Read the model definition and answer for the solid it produces. Units are mm, in the model's axes. Face numbers are marked on the shaded views. Give positions to 0.01 mm unless a question says otherwise; leave off trailing zeros. Loops run counter-clockwise (first coordinate to the right, second up) from the corner with the lowest first, then second, coordinate; pieces in that order, holes last. Notation, with made-up numbers: M -38.75,-3 L 6.25,-3 A21 ccw 6.25,4 Z; hole C 43,30.25 d7. An arc over 180 degrees is marked long. Return JSON: item names as keys, results as strings. Group by question number.
```python
from build123d import *

# Parameters (mm, degrees)
SKETCH1_R           = 28.5
SKETCH1_R_2         = 23.6
BOSS_EXTRUDE1_DEPTH = 44
SKETCH2_R           = 6
BOSS_EXTRUDE2_DEPTH = 44
SKETCH3_R           = 3.1
CUT_EXTRUDE1_DEPTH  = 45


with BuildPart() as part:
    # Sketch1 → Boss-Extrude1 (new body)
    with BuildSketch(Plane.XY):
        Circle(SKETCH1_R)
        Circle(SKETCH1_R_2, mode=Mode.SUBTRACT)
    extrude(amount=BOSS_EXTRUDE1_DEPTH)

    # Sketch2 → Boss-Extrude2 (add)
    with BuildSketch(Plane(origin=(0, 0, 0), x_dir=(-1, 0, 0), z_dir=(0, 0, -1))):
        with Locations((0, 29.6)):
            Circle(SKETCH2_R)
        with Locations((29.6, 0)):
            Circle(SKETCH2_R)
        with Locations((0, -29.6)):
            Circle(SKETCH2_R)
        with Locations((-29.6, 0)):
            Circle(SKETCH2_R)
    extrude(amount=-BOSS_EXTRUDE2_DEPTH)

    # Sketch3 → Cut-Extrude1 (cut, through all)
    with BuildSketch(Plane(origin=(0, 0, 0), x_dir=(-1, 0, 0), z_dir=(0, 0, -1))):
        with Locations((0, 29.6)):
            Circle(SKETCH3_R)
        with Locations((29.6, 0)):
            Circle(SKETCH3_R)
        with Locations((-29.6, 0)):
            Circle(SKETCH3_R)
        with Locations((0, -29.6)):
            Circle(SKETCH3_R)
    extrude(amount=-CUT_EXTRUDE1_DEPTH, mode=Mode.SUBTRACT)


solid = part.part
```
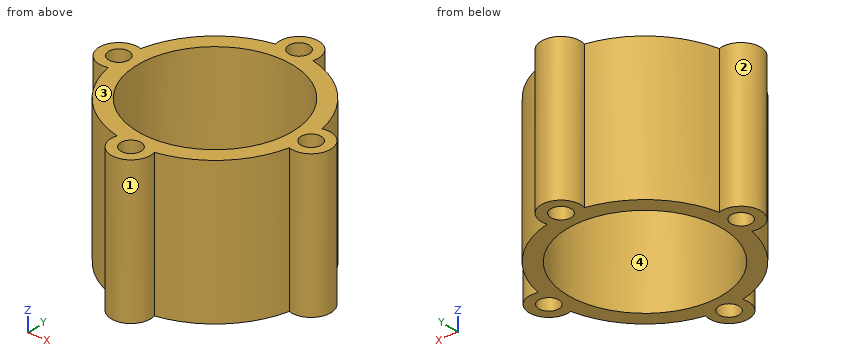
1. Find section D-D (z = 9.5). Write down the section's boundary in (x, y), and give its area (3 significant figures).
2. The mould has two halves that part along X. Classify the marked faces 1, 2, 3 and 4: +X half, -X half, draft (parallel to the pull), parting line (faces both ways), or undercut.
3. Find section B-B (y = -29.6). Write down the section's boundary in (x, z).
4. Straight lines are drawn through the part: line 1 along Y through (x, z) = (0, 25); line 2 along Y through (x, z) = (29.6, 16); line 3 along Y through (x, z) = (1, 42). For each, find the intervals that lie inside material, in ascending order.
5. Flat-ended cylindrical pins translate along their axes: P1, Ø1.5, axis at x = 7.5, z = 19, coming from the -Y side; P2, Ø12, axis at y = 23, z = 24, coming from the -X side; P3, Ø12, axis at y = -28, z = 24, coming from the +X side. Find the tip coordinate at first contact, or state that the pin passes through.
6. Find section A-A (x = 0). Write down the section's boundary in (y, z), and give its area (3 significant figures).
Result:
{
 "1": {"outline": "M -27.91,-5.76 A28.5 ccw -5.76,-27.91 A6 ccw long 5.76,-27.91 A28.5 ccw 27.91,-5.76 A6 ccw long 27.91,5.76 A28.5 ccw 5.76,27.91 A6 ccw long -5.76,27.91 A28.5 ccw -27.91,5.76 A6 ccw long Z; hole C -29.6,0 d6.2; hole C 0,0 d47.2; hole C 0,-29.6 d6.2; hole C 0,29.6 d6.2; hole C 29.6,0 d6.2", "area": "969 mm2"},
 "2": {"face 1": "parting line", "face 2": "undercut", "face 3": "draft", "face 4": "undercut"},
 "3": {"outline": "M -6,0 L -3.1,0 L -3.1,44 L -6,44 Z; M 3.1,0 L 6,0 L 6,44 L 3.1,44 Z"},
 "4": {"line 1": "y = -35.6 to -32.7, -26.5 to -23.6, 23.6 to 26.5, 32.7 to 35.6", "line 2": "y = -6 to -3.1, 3.1 to 6", "line 3": "y = -35.52 to -32.53, -26.67 to -23.58, 23.58 to 26.67, 32.53 to 35.52"},
 "5": {"P1": "stops at y = -27.69", "P2": "stops at x = -22.87", "P3": "stops at x = 18.12"},
 "6": {"outline": "M -35.6,0 L -32.7,0 L -32.7,44 L -35.6,44 Z; M -26.5,0 L -23.6,0 L -23.6,44 L -26.5,44 Z; M 23.6,0 L 26.5,0 L 26.5,44 L 23.6,44 Z; M 32.7,0 L 35.6,0 L 35.6,44 L 32.7,44 Z", "area": "510 mm2"}
}
